```python
from build123d import *

# Parameters (mm, degrees)
SKETCH_1_R      = 4
EXTRUDE_1_DEPTH = 3
SKETCH_2_R      = 5.5
SKETCH_2_R_2    = 4
EXTRUDE_2_DEPTH = 10


with BuildPart() as part:
    # 草图1 → 凸台-拉伸1 (new body)
    with BuildSketch(Plane.XY):
        with BuildLine():
            Line((-6.52657961, 5.455372618), (30.448093928, 5.455372618))
            ThreePointArc((30.448093928, 5.455372618), (44.460757159, 1.735800378), (30.448093928, -1.983771861))
            Line((30.448093928, -1.983771861), (-6.52657961, -1.983771861))
            ThreePointArc((-6.52657961, -1.983771861), (-20.539242841, 1.735800378), (-6.52657961, 5.455372618))
        make_face()
        with Locations((-13.039242841, 1.735800378)):
            Circle(SKETCH_1_R, mode=Mode.SUBTRACT)
        with Locations(Location((36.960757159, 1.735800378, 0), (0, 0, 180))):
            Circle(SKETCH_1_R, mode=Mode.SUBTRACT)
    extrude_1 = extrude(amount=EXTRUDE_1_DEPTH)

    # 草图2 → 凸台-拉伸2 (add)
    # profile 1 of 2: a face of its own
    with BuildSketch(Plane.XY.offset(3)):
        with Locations((-13.039242841, 1.735800378)):
            Circle(SKETCH_2_R)
        with Locations((-13.039242841, 1.735800378)):
            Circle(SKETCH_2_R_2, mode=Mode.SUBTRACT)
    # profile 2 of 2: a face of its own
    with BuildSketch(Plane.XY.offset(3)):
        with Locations((36.960757159, 1.735800378)):
            Circle(SKETCH_2_R)
        with Locations(Location((36.960757159, 1.735800378, 0), (0, 0, 180))):
            Circle(SKETCH_2_R_2, mode=Mode.SUBTRACT)
    extrude(amount=EXTRUDE_2_DEPTH)

    # 镜向1: 凸台-拉伸1 across plane
    add(extrude_1.mirror(Plane.XY.offset(8)))


solid = part.part
```
Can you work these out from the model? Positions are in its coordinate system, mm. A direction names the side the tool comes from. Coordinates: 2 decimals unless noted, no trailing zeros. Write each loop counter-clockwise with the first axis right and the second up, starting at its lowest first coordinate (ties: lowest second). Pieces come first, ordered by that corner, then holes. Notation, with made-up numbers: M -24.5,54 L 8.5,54 A7 ccw 8.5,62 Z; hole C 80.5,-26.5 d6. An arc over 180 degrees is marked long. Answer as CSV lines item,"result".
Item 1: We'd pull the mould along Z, two halves only. Please class faces 1 (the flat face through (12, 2, 0)), 2 (the flat face through (12, 2, 16)), 3 (the flat face through (12, 2, 13)), 4 (the cylindrical face through (44.456, 2.011, 1.479)): +Z half, -Z half, draft (parallel to the pull), parting line (faces both ways), or undercut.
Geometry results:
face 1,"-Z half"
face 2,"+Z half"
face 3,"undercut"
face 4,"draft"
Item 2: Imagine slicing it at D-D on z = 15.25. List the corners of the cut face in (x, y) for me.
Geometry results:
outline,"M -6.53,-1.98 L 30.45,-1.98 A7.5 ccw long 30.45,5.46 L -6.53,5.46 A7.5 ccw long Z; hole C -13.04,1.74 d8; hole C 36.96,1.74 d8"
Item 3: On a 3-axis mill with a long thin cutter (end or side, diameter ignored), from which of +Z, -Z, +X, -X, +Y, -Y can I reach the whole of each face in a straight line? I mean faces 5 (the cylindrical face through (-17.093, 5.453, 7.93)), 6 (the flat face through (12, 5.455, 15)), 7 (the cylindrical face through (40.135, 4.17, 8.112)), 8 (the flat face through (12, -1.984, 15)). Say none if no direction works.
Geometry results:
face 5,"none"
face 6,"+Z, -Z, +Y"
face 7,"+Z, -Z"
face 8,"+Z, -Z, -Y"
Item 4: Please list where these lines run through material, in increasing order: line 1 along X through (y, z) = (2.5, 14.5); line 2 along Z through (x, y) = (34.5, 7.75); line 3 along X through (y, z) = (4.75, 15).
Geometry results:
line 1,"x = -20.5 to -16.97, -9.11 to 33.03, 40.89 to 44.42"
line 2,"z = 0 to 3, 13 to 16"
line 3,"x = -19.91 to -15.67, -10.41 to 34.33, 39.59 to 43.83"
Item 5: Imagine slicing it at B-B on x = 25. List the corners of the cut face in (y, z) for me, plus the area to 3 significant figures.
Geometry results:
outline,"M -1.98,0 L 5.46,0 L 5.46,3 L -1.98,3 Z; M -1.98,13 L 5.46,13 L 5.46,16 L -1.98,16 Z"
area,"44.6 mm2"
Item 6: Imagine slicing it at A-A on y = -1. List the corners of the cut face in (x, z) for me, plus the area to 3 significant figures.
Geometry results:
outline,"M -20.02,0 L -15.96,0 L -15.96,16 L -20.02,16 L -20.02,13 L -17.81,13 L -17.81,3 L -20.02,3 Z; M -10.12,0 L 34.04,0 L 34.04,16 L -10.12,16 Z; M 39.88,0 L 43.94,0 L 43.94,3 L 41.73,3 L 41.73,13 L 43.94,13 L 43.94,16 L 39.88,16 Z; hole M -8.27,3 L 32.19,3 L 32.19,13 L -8.27,13 Z"
area,"388 mm2"
Item 7: I'm going to push flat-ended pins straight in: P1, Ø4, axis at y = -2, z = 13.5, coming from the +X side; P2, Ø0.9, axis at x = 15.5, z = 1.5, coming from the -Y side; P3, Ø1.5, axis at x = -11.5, z = 13.5, coming from the +Y side. Where does each tip first touch, or does it pass through?
Geometry results:
P1,"stops at x = 44.26"
P2,"stops at y = -1.98"
P3,"stops at y = 9.19"
Item 8: Imagine slicing it at C-C on y = 8.25. List the corners of the cut face in (x, z) for me, plus the area to 3 significant figures.
Geometry results:
outline,"M -16.76,0 L -9.32,0 L -9.32,3 L -16.76,3 Z; M -16.76,13 L -9.32,13 L -9.32,16 L -16.76,16 Z; M 33.24,0 L 40.68,0 L 40.68,3 L 33.24,3 Z; M 33.24,13 L 40.68,13 L 40.68,16 L 33.24,16 Z"
area,"89.2 mm2"
